Build history of the part. All positions in model axes, mm. Face numbers are marked on the shaded views. A direction names the side the tool comes from. Coordinates: 2 decimals unless noted, no trailing zeros. Order: outer loops, then holes, each group sorted by start corner. A loop starts at its lowest first (then second) coordinate and runs counter-clockwise, first axis right, second up. Notation, with made-up numbers: (40, 84) - (85, 84) arc R16 cw to (85, 97) - close; hole circle Ø3 at (16.5, 11). An arc over 180 degrees is marked (long way). One line per item, written item: value.
from build123d import *

# Parameters (mm, degrees)
F1_R     = 15
F2_DEPTH = 2.5


with BuildPart() as f2:
    # F1 (on Front) → F2 (new body)
    with BuildSketch(Plane.XZ):
        with Locations((10, 5)):
            Circle(F1_R)
        Polygon((4.375, 0.625), (0, 5), (5, 5), (5, 10), (9.375, 5.625), align=None, mode=Mode.SUBTRACT)
        Polygon((15, 0), (5, 0), (15, 10), (15, 5), (20, 5), align=None, mode=Mode.SUBTRACT)
    extrude(amount=F2_DEPTH)


solid = f2.part
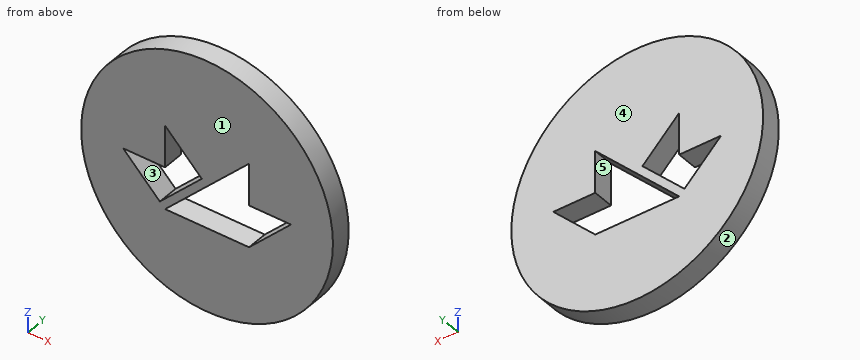
1. Band-saw the part on C-C, the plane z = 4.5. Give the cut face in (x, y).
Values found:
outline: (-4.99, -2.5) - (0.5, -2.5) - (0.5, 0) - (-4.99, 0) - close; (8.25, -2.5) - (9.5, -2.5) - (9.5, 0) - (8.25, 0) - close; (19.5, -2.5) - (24.99, -2.5) - (24.99, 0) - (19.5, 0) - close
2. 3-axis set-ups, long thin cutter, end or side, ignore diameter. For the marked faces 4 and 5: which of +Z, -Z, +X, -X, +Y, -Y reach the whole face in a straight line?
Values found:
face 4: +Z, -Z, +X, -X, +Y
face 5: +Y, -Y
3. Band-saw the part on A-A, the plane x = 10. Give the cut face in (y, z).
Values found:
outline: (-2.5, -10) - (0, -10) - (0, 0) - (-2.5, 0) - close; (-2.5, 5) - (0, 5) - (0, 20) - (-2.5, 20) - close
4. Two-plate mould, pull along X, no slides. Class the marked faces 1, 2 and 3: pulls with the +X half, pulls with the -X half, needs draft (parallel to the pull), parting line crosses it, or undercut.
Values found:
face 1: needs draft
face 2: parting line crosses it
face 3: undercut
5. Flat gauge pins, fed straight in: P1, Ø2, axis at x = 9, z = 1.5, coming from the -Y side; P2, Ø1.2, axis at x = 17.5, y = -1.5, coming from the -Z side; P3, Ø0.8, axis at x = 2.5, y = -1, coming from the -Z side. Where does each tip first touch, or does it go through?
Values found:
P1: passes through
P2: stops at z = -8.32
P3: stops at z = -8.21
6. Band-saw the part on B-B, the plane y = -1.85. Give the cut face in (x, z) (3 decimals), and give its area (3 significant figures).
Values found:
outline: circle Ø30 at (10, 5); hole (0, 5) - (4.375, 0.625) - (9.375, 5.625) - (5, 10) - (5, 5) - close; hole (5, 0) - (15, 0) - (20, 5) - (15, 5) - (15, 10) - close
area: 613 mm2
7. Probe line 1 along Z through (x, y) = (7.75, -0.25); line 2 along X through (y, z) = (-1.5, 7.25); line 3 along Z through (x, y) = (9, -1.95). List the from-to ranges inside material, lowest first.
Values found:
line 1: z = -9.83 to 0, 2.75 to 4, 7.25 to 19.83
line 2: x = -4.83 to 5, 7.75 to 12.25, 15 to 24.83
line 3: z = -9.97 to 0, 4 to 5.25, 6 to 19.97
8. Band-saw the part on D-D, the plane x = 19.5. Give the cut face in (y, z), and give its area (3 significant figures).
Values found:
outline: (-2.5, -6.61) - (0, -6.61) - (0, 4.5) - (-2.5, 4.5) - close; (-2.5, 5) - (0, 5) - (0, 16.61) - (-2.5, 16.61) - close
area: 56.8 mm2
